Input: part model. Units: mm. Frame: model coordinates. Round coordinates to 2 decimals unless told otherwise and drop trailing zeros. Loops run counter-clockwise (first coordinate to the right, second up) from the corner with the lowest first, then second, coordinate; pieces in that order, holes last. Notation, with made-up numbers: (33.5, 28.5) -> (77.5, 28.5) arc R14 cw to (77.5, 32.5) -> close; hole circle Ø3 at (72, 60.5). An arc over 180 degrees is marked (long way). Answer as a JSON object with one key per item and string values.
```python
from build123d import *

# Parameters (mm, degrees)
F0_R          = 17.5
F1_DEPTH      = 200
F2_R          = 2.5
F3_DEPTH      = 25
F3_DEPTH_BACK = 25
F4_R          = 13.5
F5_DEPTH      = 1022


with BuildPart() as f1:
    # F0 (on Top) → F1 (new body)
    with BuildSketch(Plane.XY):
        Circle(F0_R)
    extrude(amount=F1_DEPTH)

    # F2 (on Front) → F3 (cut, two sides)
    with BuildSketch(Plane.XZ) as f3_sk:
        with Locations((0, 170)):
            Circle(F2_R)
    extrude(amount=-F3_DEPTH, mode=Mode.SUBTRACT)
    extrude(f3_sk.sketch, amount=F3_DEPTH_BACK, mode=Mode.SUBTRACT)

    # F4 (on face) → F5 (cut)
    with BuildSketch(Plane.XY.offset(200)):
        Circle(F4_R)
    extrude(amount=-F5_DEPTH, mode=Mode.SUBTRACT)


solid = f1.part
```
1) Ray query, probe 1 along X at (y, z) = (-1, 171); probe 2 along Y at (x, z) = (0, 103.5); probe 3 along Z at (x, y) = (0, -15.15). Return the intervals inside material, ascending.
Output:
{"probe 1": "x = -17.47 to -13.46, 13.46 to 17.47", "probe 2": "y = -17.5 to -13.5, 13.5 to 17.5", "probe 3": "z = 0 to 167.5, 172.5 to 200"}
2) Contact query for flat-ended pins moving along their axis: P1, Ø8, axis at y = 11.5, z = 68.5, coming from the +X side; P2, Ø1.5, axis at x = 0.5, z = 87, coming from the -Y side; P3, Ø1.5, axis at x = 8, z = 72, coming from the +Y side; P4, Ø12, axis at x = 4, y = 0, coming from the -Z side. Output: stop coordinate, or through.
Output:
{"P1": "stops at x = 15.81", "P2": "stops at y = -17.5", "P3": "stops at y = 15.93", "P4": "passes through"}
3) Section C-C, the plane z = 170. Output: boundary loops of the cut face in (x, y).
Output:
{"outline": "(-2.5, -17.32) -> (-2.5, -13.27) arc R13.5 cw to (-2.5, 13.27) -> (-2.5, 17.32) arc R17.5 ccw to start; (2.5, -17.32) arc R17.5 ccw to (2.5, 17.32) -> (2.5, 13.27) arc R13.5 cw to (2.5, -13.27) -> close"}
4) Section A-A, the plane y = 0. Output: boundary loops of the cut face in (x, z), plus the area to 3 significant figures.
Output:
{"outline": "(-17.5, 0) -> (-13.5, 0) -> (-13.5, 200) -> (-17.5, 200) -> close; (13.5, 0) -> (17.5, 0) -> (17.5, 200) -> (13.5, 200) -> close", "area": "1,600 mm^2"}
5) Section D-D, the plane z = 36. Output: boundary loops of the cut face in (x, y).
Output:
{"outline": "circle Ø35 at (0, 0); hole circle Ø27 at (0, 0)"}
6) Section B-B, the plane x = 0. Output: boundary loops of the cut face in (y, z).
Output:
{"outline": "(-17.5, 0) -> (-13.5, 0) -> (-13.5, 167.5) -> (-17.5, 167.5) -> close; (-17.5, 172.5) -> (-13.5, 172.5) -> (-13.5, 200) -> (-17.5, 200) -> close; (13.5, 0) -> (17.5, 0) -> (17.5, 167.5) -> (13.5, 167.5) -> close; (13.5, 172.5) -> (17.5, 172.5) -> (17.5, 200) -> (13.5, 200) -> close"}
7) Draft query along X for faces 1 (the face through (-0.33, -15.41, 172.48)), 2 (the face through (9, -10.3, 0)), 3 (the face through (-13.887, -10.648, 98.6)), 4 (the face through (2.385, 15.353, 170.751)). Return one class per face: +X half, -X half, draft (parallel to the pull), parting line (faces both ways), or undercut.
Output:
{"face 1": "undercut", "face 2": "draft", "face 3": "parting line", "face 4": "undercut"}
